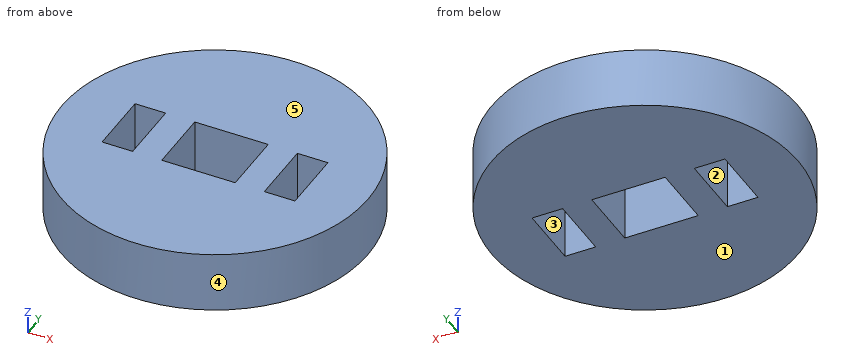
from build123d import *

# Parameters (mm, degrees)
F0_R     = 50
F0_W     = 10
F0_H     = 21
F0_W_2   = 24
F1_DEPTH = 20


with BuildPart() as f1:
    # F0 (on Top) → F1 (new body)
    with BuildSketch(Plane.XY):
        Circle(F0_R)
        with Locations((-26.5, 0)):
            Rectangle(F0_W, F0_H, mode=Mode.SUBTRACT)
        Rectangle(F0_W_2, F0_H, mode=Mode.SUBTRACT)
        with Locations((26.5, 0)):
            Rectangle(F0_W, F0_H, mode=Mode.SUBTRACT)
    extrude(amount=-F1_DEPTH)


solid = f1.part
Verification items for the finished model (mm, model axes). Face numbers are marked on the shaded views. A direction names the side the tool comes from. Coordinates: 2 decimals unless noted, no trailing zeros. Order: outer loops, then holes, each group sorted by start corner. A loop starts at its lowest first (then second) coordinate and runs counter-clockwise, first axis right, second up. Notation, with made-up numbers: M 11.25,69 L 17.25,69 A14 cw 17.25,80 Z; hole C 26.5,-6.5 d5. An arc over 180 degrees is marked long. One line per item, written item: value. Start each with the question number.
Item 1: Sectioned sample at D-D on x = -36. Record the cut outline in (y, z).
Item 2: Sectioned sample at A-A on x = 0. Record the cut outline in (y, z), then the cut area to 3 significant figures.
Item 3: Sectioned sample at B-B on y = 0. Record the cut outline in (x, z).
Item 4: Sectioned sample at C-C on z = -9.5. Record the cut outline in (x, y), then the cut area to 3 significant figures.
Item 5: Thickness scan on probe 1 along X at (y, z) = (-6.5, -13); probe 2 along Y at (x, z) = (29.5, -9.5); probe 3 along Y at (x, z) = (-10, -4.25). Record the ranges inside material, lowest first.
Item 6: Depth check by flat-ended pin: P1, Ø1, axis at x = -2, z = -12.5, coming from the -Y side; P2, Ø5, axis at x = 24.5, z = -5.5, coming from the +Y side; P3, Ø11, axis at x = -24, z = -6.5, coming from the +Y side. Enter the tip coordinate at first touch or a pass-through.
Item 7: Mould release check, pull along X, two halves, no side actions. Record for the marked faces 3, 4 and 5: pulls with the +X half, pulls with the -X half, needs draft (parallel to the pull), parting line crosses it, or undercut.
Item 8: Access from +Z, -Z, +X, -X, +Y, -Y to the whole of each face (thin tool, end or side, straight path). Record for the marked faces 1 and 2.
Calculated:
1. outline: M -34.7,-20 L 34.7,-20 L 34.7,0 L -34.7,0 Z
2. outline: M -50,-20 L -10.5,-20 L -10.5,0 L -50,0 Z; M 10.5,-20 L 50,-20 L 50,0 L 10.5,0 Z
2. area: 1,580 mm^2
3. outline: M -50,-20 L -31.5,-20 L -31.5,0 L -50,0 Z; M -21.5,-20 L -12,-20 L -12,0 L -21.5,0 Z; M 12,-20 L 21.5,-20 L 21.5,0 L 12,0 Z; M 31.5,-20 L 50,-20 L 50,0 L 31.5,0 Z
4. outline: C 0,0 d100; hole M -31.5,-10.5 L -21.5,-10.5 L -21.5,10.5 L -31.5,10.5 Z; hole M -12,-10.5 L 12,-10.5 L 12,10.5 L -12,10.5 Z; hole M 21.5,-10.5 L 31.5,-10.5 L 31.5,10.5 L 21.5,10.5 Z
4. area: 6,930 mm^2
5. probe 1: -49.58 to -31.5, -21.5 to -12, 12 to 21.5, 31.5 to 49.58
5. probe 2: -40.37 to -10.5, 10.5 to 40.37
5. probe 3: -48.99 to -10.5, 10.5 to 48.99
6. P1: y = -49.98
6. P2: y = 44.9
6. P3: y = 46.45
7. face 3: undercut
7. face 4: parting line crosses it
7. face 5: needs draft
8. face 1: -Z, +X, -X, +Y, -Y
8. face 2: +Z, -Z
